Input: part model. Units: mm. Frame: model coordinates. Coordinates: 2 decimals unless noted, no trailing zeros. Order: outer loops, then holes, each group sorted by start corner. A loop starts at its lowest first (then second) coordinate and runs counter-clockwise, first axis right, second up. Notation, with made-up numbers: (53.25, 17.25) - (112.25, 17.25) arc R17 cw to (112.25, 46.25) - close; hole circle Ø9 at (-13.5, 34). An arc over 180 degrees is marked (long way). Answer as CSV lines item,"result". Start each with the question number.
Item 1: Material intervals for line 1 along Z through (x, y) = (-59, 7.75); line 2 along Z through (x, y) = (-57.5, 2.5); line 3 along X through (y, z) = (2.5, 45), sorted ascending.
Item 2: Section B-B (z = -26). Output: boundary loops of the cut face in (x, y).
Item 3: Draft query along Z for faces 1 (the flat face through (-64, 9, -27)), 2 (the cylindrical face through (65.586, 4.437, 27.193)), 3 (the cylindrical face through (63.738, 4.437, 26.427)). Return one class per face: +Z half, -Z half, draft (parallel to the pull), parting line (faces both ways), or undercut.
Item 4: First-contact query: pin 1 (0.6 mm diameter, centred on x = -50, z = 49.5, fed in from +Y); pin 2 (0.5 mm diameter, centred on x = -70, z = 0, fed in from +Y); pin 3 (1 mm diameter, centred on y = 5, z = -18.5, fed in from +X); pin 4 (1 mm diameter, centred on y = 7.5, z = -20.5, fed in from -X). Flat tips, straight axial feed; report the tip coordinate or a pass-through.
Item 5: Section A-A (y = 5.5). State how many separate pieces and enclosed holes the cut face has, and give its area (3 significant figures).
from build123d import *

# Parameters (mm, degrees)
SKETCH1_R           = 71
SKETCH1_R_2         = 69
BOSS_EXTRUDE1_DEPTH = 9
CUT_EXTRUDE1_DEPTH  = 7
CIRPATTERN1_COUNT   = 8


with BuildPart() as part:
    # Sketch1 → Boss-Extrude1 (new body)
    with BuildSketch(Plane(origin=(0, 0, 0), x_dir=(1, 0, 0), z_dir=(0, 1, 0))):
        Circle(SKETCH1_R)
        Circle(SKETCH1_R_2, mode=Mode.SUBTRACT)
    extrude(amount=BOSS_EXTRUDE1_DEPTH)

    # Sketch2 → Cut-Extrude1 (cut)
    with BuildSketch(Plane(origin=(0, 9, 0), x_dir=(1, 0, 0), z_dir=(0, 1, 0))):
        with BuildLine():
            Line((0.5, 68.998188382), (0.5, 70.998239415))
            ThreePointArc((0.5, 70.998239415), (0, 71), (-0.5, 70.998239415))
            Line((-0.5, 70.998239415), (-0.5, 68.998188382))
            ThreePointArc((-0.5, 68.998188382), (0, 69), (0.5, 68.998188382))
        make_face()
    cut_extrude1 = extrude(amount=-CUT_EXTRUDE1_DEPTH, mode=Mode.SUBTRACT)

    # CirPattern1: Cut-Extrude1 ×8 about axis
    cirpattern1_axis = Axis((0, 0, 0), (0, 1, 0))
    for i in range(1, CIRPATTERN1_COUNT):
        add(cut_extrude1.rotate(cirpattern1_axis, i * 360 / CIRPATTERN1_COUNT), mode=Mode.SUBTRACT)


solid = part.part
Determined:
1,line 1,"z = -39.5 to -35.78, 35.78 to 39.5"
1,line 2,"z = -41.65 to -38.14, 38.14 to 41.65"
1,line 3,"x = -54.92 to -52.31, 52.31 to 54.92"
2,outline,"(-66.07, 0) - (-63.91, 0) - (-63.91, 9) - (-66.07, 9) - close; (63.91, 0) - (66.07, 0) - (66.07, 9) - (63.91, 9) - close"
3,face 1,"draft"
3,face 2,"parting line"
3,face 3,"undercut"
4,pin 1,"stops at y = 9"
4,pin 2,"stops at y = 2"
4,pin 3,"stops at x = 68.68"
4,pin 4,"stops at x = -68.12"
5,separate pieces,"8"
5,enclosed holes,"0"
5,area,"864 mm^2"
